Read the model definition and answer for the solid it produces. Units are mm, in the model's axes. Round coordinates to 2 decimals unless told otherwise and drop trailing zeros. Loops run counter-clockwise (first coordinate to the right, second up) from the corner with the lowest first, then second, coordinate; pieces in that order, holes last. Notation, with made-up numbers: M 1.25,51 L 43.25,51 A34 ccw 43.25,89 Z; hole C 81.25,53.5 d4. An arc over 180 degrees is marked long. Write each question's results on one line, items separated by ' | '.
from build123d import *

# Parameters (mm, degrees)
SKETCH8_W                      = 120
SKETCH8_H                      = 150
BOSS_EXTRUDE3_DEPTH            = 5
SKETCH9_R                      = 50
BOSS_EXTRUDE4_DEPTH            = 5
BOSS_EXTRUDE8_OUTLINE_R        = 5.460321951
BOSS_EXTRUDE8_DEPTH            = 1
CUT_EXTRUDE9_OUTLINE_R         = 5
CUT_EXTRUDE9_DEPTH             = 3
F_2_0_221_DIAMETER_HOLE1_D     = 5.6134
F_2_0_221_DIAMETER_HOLE1_DEPTH = 8
F_2_0_221_DIAMETER_HOLE1_TIP   = 1.686435499
FILLET3_R                      = 4
SKETCH38_W                     = 26
SKETCH38_H                     = 70
CUT_EXTRUDE10_DEPTH            = 40
SKETCH39_W                     = 25
SKETCH39_H                     = 18
CUT_EXTRUDE11_DEPTH            = 40
DRAFT1_ANGLE                   = 1
DRAFT2_ANGLE                   = 1


# Read off the part's stored shape, not the designer's step: Boss-Extrude8, Cut-Extrude9, Draft5, Draft6
with BuildPart() as part:
    # Sketch8 → Boss-Extrude3 (new body)
    with BuildSketch(Plane(origin=(0, 0, 0), x_dir=(1, 0, 0), z_dir=(0, 1, 0))):
        with Locations((73.708855083, 72.164227744)):
            Rectangle(SKETCH8_W, SKETCH8_H)
    extrude(amount=BOSS_EXTRUDE3_DEPTH)

    # Sketch9 → Boss-Extrude4 (add)
    with BuildSketch(Plane(origin=(0, 0, 0), x_dir=(1, 0, 0), z_dir=(0, 1, 0))):
        with Locations((-22.779007595, 71.748458752)):
            Circle(SKETCH9_R)
    extrude(amount=BOSS_EXTRUDE4_DEPTH)

    # Boss-Extrude8 outline → Boss-Extrude8 (cut)
    with BuildSketch(Plane(origin=(0, 0, 0), x_dir=(1, 0, 0), z_dir=(0, 1, 0))):
        with Locations((19.708855083, 3.164227744)):
            Circle(BOSS_EXTRUDE8_OUTLINE_R)
    extrude(amount=BOSS_EXTRUDE8_DEPTH, mode=Mode.SUBTRACT)

    # Cut-Extrude9 outline → Cut-Extrude9 (cut)
    with BuildSketch(Plane(origin=(0, 0, 0), x_dir=(1, 0, 0), z_dir=(0, 1, 0))):
        with Locations((127.708855083, 141.164227744)):
            Circle(CUT_EXTRUDE9_OUTLINE_R)
    extrude(amount=CUT_EXTRUDE9_DEPTH, mode=Mode.SUBTRACT)

    # #2 (0.221) Diameter Hole1
    with Locations(Plane(origin=(0, 5, 0), x_dir=(1, 0, 0), z_dir=(0, 1, 0))):
        with Locations((18.917123201, 141.531370062), (127.969984407, 141.269223761), (127.602547564, 3.45328248), (19.774147178, 3.570575466), (-67.115618064, 71.668740496)):
            Hole(F_2_0_221_DIAMETER_HOLE1_D / 2, depth=F_2_0_221_DIAMETER_HOLE1_DEPTH)
            with Locations((0, 0, -(F_2_0_221_DIAMETER_HOLE1_DEPTH + F_2_0_221_DIAMETER_HOLE1_TIP / 2))):  # 118° drill point
                Cone(0, F_2_0_221_DIAMETER_HOLE1_D / 2, F_2_0_221_DIAMETER_HOLE1_TIP, mode=Mode.SUBTRACT)

    # Fillet3
    fillet3_edges = [part.edges().sort_by_distance(p)[0] for p in [
        (13.708855083, 2.5, -147.164227744),
        (133.708855083, 2.5, -147.164227744),
        (133.708855083, 2.5, 2.835772256),
        (13.708855083, 2.5, 2.835772256),
    ]]
    fillet(fillet3_edges, radius=FILLET3_R)

    # Sketch38 → Cut-Extrude10 (cut)
    with BuildSketch(Plane(origin=(0, 5, 0), x_dir=(1, 0, 0), z_dir=(0, 1, 0))):
        with Locations((-21.291144917, 72.164227744)):
            Rectangle(SKETCH38_W, SKETCH38_H)
    extrude(amount=-CUT_EXTRUDE10_DEPTH, mode=Mode.SUBTRACT)

    # Sketch39 → Cut-Extrude11 (cut)
    with BuildSketch(Plane(origin=(0, 5, 0), x_dir=(1, 0, 0), z_dir=(0, 1, 0))):
        with Locations((44.875898376, 128.991672485)):
            Rectangle(SKETCH39_W, SKETCH39_H)
    extrude(amount=-CUT_EXTRUDE11_DEPTH, mode=Mode.SUBTRACT)

    # Draft1
    draft1_faces = [part.faces().sort_by_distance(p)[0] for p in [
        (130.409247564, 2.5, -3.45328248),
        (132.537282207, 2.5, 1.664199381),
        (73.708855083, 2.5, 2.835772256),
        (44.875898376, 2.5, -137.991672485),
        (-21.291144917, 2.5, -107.164227744),
        (14.880427958, 2.5, 1.664199381),
        (57.375898376, 2.5, -128.991672485),
        (-34.291144917, 2.5, -72.164227744),
        (32.375898376, 2.5, -128.991672485),
        (133.708855083, 2.5, -72.164227744),
        (130.776684407, 4, -141.269223761),
        (132.537282207, 2.5, -145.992654868),
        (13.708855083, 2.5, -19.363684902),
        (22.580847178, 3, -3.570575466),
        (13.708855083, 2.5, -124.549001593),
        (-8.291144917, 2.5, -72.164227744),
        (-64.308918064, 2.5, -71.668740496),
        (-21.291144917, 2.5, -37.164227744),
        (-72.779007595, 2.5, -71.748458752),
        (21.723823201, 2.5, -141.531370062),
        (14.880427958, 2.5, -145.992654868),
        (44.875898376, 2.5, -119.991672485),
        (73.708855083, 2.5, -147.164227744),
    ]]
    draft(draft1_faces, Plane.ZX.offset(5), DRAFT1_ANGLE)

    # Draft2
    draft2_faces = [part.faces().sort_by_distance(p)[0] for p in [
        (14.248533132, 0.5, -3.164227744),
        (122.708855083, 1.5, -141.164227744),
    ]]
    draft(draft2_faces, Plane(origin=(0, 0, 0), x_dir=(0, 0, -1), z_dir=(0, -1, 0)), DRAFT2_ANGLE)

    # Draft5 outline → Draft5 (revolve)
    with BuildSketch(Plane(origin=(19.708855083, 0, -3.164227744), x_dir=(1, 0, 0), z_dir=(0, 0, 1))):
        Polygon((5.303226367, 1), (5.285771302, 0), (5.460321951, 0), (5.442866886, 1), align=None)
    revolve(axis=Axis((19.708855083, 0, -3.164227744), (0, 1, 0)))

    # Draft6 outline → Draft6 (revolve)
    with BuildSketch(Plane(origin=(127.708855083, 0, -141.164227744), x_dir=(1, 0, 0), z_dir=(0, 0, 1))):
        Polygon((4.877814546, 3), (4.825449351, 0), (5, 0), (4.947634805, 3), align=None)
    revolve(axis=Axis((127.708855083, 0, -141.164227744), (0, 1, 0)))


solid = part.part
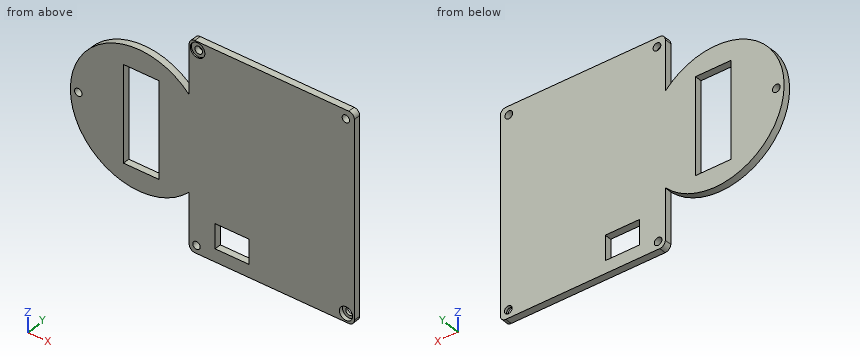
Item 1: The part is cut by section B-B (y = 1.85). Determine the outline of the cut face in (x, z).
Outcome:
outline: M 13.65,-143.16 A4.05 ccw 17.71,-147.22 L 129.71,-147.22 A4.05 ccw 133.76,-143.16 L 133.76,-1.16 A4.05 ccw 129.71,2.89 L 17.71,2.89 A4.05 ccw 13.65,-1.16 L 13.65,-37.42 A50.05 ccw long 13.65,-106.07 Z; hole C -67.12,-71.67 d5.5; hole M -34.24,-107.11 L -8.35,-107.11 L -8.35,-37.22 L -34.24,-37.22 Z; hole C 18.92,-141.53 d5.5; hole C 19.77,-3.57 d5.5; hole M 32.43,-137.94 L 57.32,-137.94 L 57.32,-120.05 L 32.43,-120.05 Z; hole C 127.71,-141.16 d9.72; hole C 127.6,-3.45 d5.5
Item 2: Straight lines are drawn through the part: line 1 (Z direction, x = -21, y = 0.2); line 2 (X direction, y = 4.6, z = -126); line 3 (X direction, y = 1.3, z = -140). For each, find the intervals that lie inside material, in ascending order.
Outcome:
line 1: z = -121.8 to -107.08, -37.25 to -21.7 | line 2: x = 13.7 to 32.38, 57.37 to 133.72 | line 3: x = 13.64 to 16.64, 21.19 to 123, 132.42 to 133.77
Item 3: The part is cut by section A-A (z = -127.5). Determine the outline of the cut face in (x, y), plus the area to 3 significant figures.
Outcome:
outline: M 13.62,0 L 32.46,0 L 32.38,5 L 13.71,5 Z; M 57.29,0 L 133.8,0 L 133.71,5 L 57.38,5 Z | area: 476 mm2
Item 4: Flat-ended cylindrical pins translate along their axes: pin 1 (1.5 mm diameter, centred on x = 50.5, y = 4.5, fed in from +Z); pin 2 (2 mm diameter, centred on y = 3.5, z = -91.5, fed in from -X); pin 3 (5.5 mm diameter, centred on x = 20.5, z = -2.5, fed in from -Y). Find the tip coordinate at first contact, or state that the pin passes through.
Outcome:
pin 1: stops at z = 2.86 | pin 2: stops at x = -69.16 | pin 3: stops at y = 1
